Part model, mm, in its own coordinate system. A direction names the side the tool comes from. Give positions to 0.01 mm unless a question says otherwise; leave off trailing zeros. Loops run counter-clockwise (first coordinate to the right, second up) from the corner with the lowest first, then second, coordinate; pieces in that order, holes last. Notation, with made-up numbers: (80, 34.5) -> (90, 34.5) arc R12 cw to (90, 43.5) -> close; hole circle Ø8 at (-19.75, -17). An arc over 180 degrees is marked (long way). One line per question, with ' | ' between items.
```python
from build123d import *

# Parameters (mm, degrees)
PAD009_START    = 5
SKETCH014_R     = 1.4
SKETCH014_W     = 4
SKETCH014_H     = 8
SKETCH014_W_2   = 8
SKETCH014_H_2   = 4
PAD009_DEPTH    = 5
POCKET010_DEPTH = 2.5
POCKET011_DEPTH = 3
SKETCH022_R     = 2.5
POCKET012_DEPTH = 1
POCKET012_TAPER = 45


with BuildPart() as part:
    # Sketch014 → Pad009 (new body)
    with BuildSketch(Plane.XY.offset(PAD009_START)):
        with BuildLine():
            Line((-89, 43), (-89, -43))
            ThreePointArc((-89, -43), (-87.535534, -46.535534), (-84, -48))
            Line((-84, -48), (31, -48))
            ThreePointArc((31, -48), (34.535534, -46.535534), (36, -43))
            Line((36, -43), (36, 43))
            ThreePointArc((36, 43), (34.535534, 46.535534), (31, 48))
            Line((31, 48), (-84, 48))
            ThreePointArc((-84, 48), (-87.535534, 46.535534), (-89, 43))
        make_face()
        with Locations((-9, 43)):
            Circle(SKETCH014_R, mode=Mode.SUBTRACT)
        with Locations((9, 43)):
            Circle(SKETCH014_R, mode=Mode.SUBTRACT)
        with Locations((-9, -43)):
            Circle(SKETCH014_R, mode=Mode.SUBTRACT)
        with Locations((9, -43)):
            Circle(SKETCH014_R, mode=Mode.SUBTRACT)
        with Locations((-37.5, 12)):
            Circle(SKETCH014_R, mode=Mode.SUBTRACT)
        with Locations((2.5, 12)):
            Circle(SKETCH014_R, mode=Mode.SUBTRACT)
        with Locations((2.5, -12)):
            Circle(SKETCH014_R, mode=Mode.SUBTRACT)
        with Locations((-37.5, -12)):
            Circle(SKETCH014_R, mode=Mode.SUBTRACT)
        with Locations((-83.5, 15)):
            Circle(SKETCH014_R, mode=Mode.SUBTRACT)
        with Locations((-63.5, 15)):
            Circle(SKETCH014_R, mode=Mode.SUBTRACT)
        with Locations((-63.5, -15)):
            Circle(SKETCH014_R, mode=Mode.SUBTRACT)
        with Locations((-83.5, -15)):
            Circle(SKETCH014_R, mode=Mode.SUBTRACT)
        with Locations((-46.5, 24.5)):
            Circle(SKETCH014_R, mode=Mode.SUBTRACT)
        with Locations((-46.5, -24.5)):
            Circle(SKETCH014_R, mode=Mode.SUBTRACT)
        with Locations((11.5, -24.5)):
            Circle(SKETCH014_R, mode=Mode.SUBTRACT)
        with Locations((11.5, 24.5)):
            Circle(SKETCH014_R, mode=Mode.SUBTRACT)
        with BuildLine():
            Line((-9, 35), (-9, 29))
            ThreePointArc((-9, 29), (-8.707107, 28.292893), (-8, 28))
            Line((-8, 28), (8, 28))
            ThreePointArc((8, 28), (8.707107, 28.292893), (9, 29))
            Line((9, 29), (9, 35))
            ThreePointArc((9, 35), (8.707107, 35.707107), (8, 36))
            Line((8, 36), (-8, 36))
            ThreePointArc((-8, 36), (-8.707107, 35.707107), (-9, 35))
        make_face(mode=Mode.SUBTRACT)
        with BuildLine():
            Line((-9, -29), (-9, -35))
            ThreePointArc((-9, -35), (-8.707107, -35.707107), (-8, -36))
            Line((-8, -36), (8, -36))
            ThreePointArc((8, -36), (8.707107, -35.707107), (9, -35))
            Line((9, -35), (9, -29))
            ThreePointArc((9, -29), (8.707107, -28.292893), (8, -28))
            Line((8, -28), (-8, -28))
            ThreePointArc((-8, -28), (-8.707107, -28.292893), (-9, -29))
        make_face(mode=Mode.SUBTRACT)
        Polygon((28.8, 45), (28.8, 37), (21.9, 37), (21.9, 37.6), (15, 37.6), (15, 44.4), (21.9, 44.4), (21.9, 45), align=None, mode=Mode.SUBTRACT)
        with Locations((32, 29)):
            Rectangle(SKETCH014_W, SKETCH014_H, mode=Mode.SUBTRACT)
        with Locations((32, -29)):
            Rectangle(SKETCH014_W, SKETCH014_H, mode=Mode.SUBTRACT)
        with Locations((-29, 44)):
            Rectangle(SKETCH014_W_2, SKETCH014_H_2, mode=Mode.SUBTRACT)
        with Locations((-29, -44)):
            Rectangle(SKETCH014_W_2, SKETCH014_H_2, mode=Mode.SUBTRACT)
        with Locations((-85, 29)):
            Rectangle(SKETCH014_W, SKETCH014_H, mode=Mode.SUBTRACT)
        with Locations((-85, -29)):
            Rectangle(SKETCH014_W, SKETCH014_H, mode=Mode.SUBTRACT)
    extrude(amount=PAD009_DEPTH)

    # Sketch020 (on Face73 of Pad009) → Pocket010 (cut)
    with BuildSketch(Plane(origin=(0, 0, 5), x_dir=(1, 0, 0), z_dir=(0, 0, -1))):
        Polygon((-46.5, -27.5), (-43.901924, -26), (-43.901924, -23), (-46.5, -21.5), (-49.098076, -23), (-49.098076, -26), align=None)
        Polygon((-46.5, 27.5), (-49.098076, 26), (-49.098076, 23), (-46.5, 21.5), (-43.901924, 23), (-43.901924, 26), align=None)
        Polygon((11.5, 27.5), (8.901924, 26), (8.901924, 23), (11.5, 21.5), (14.098076, 23), (14.098076, 26), align=None)
        Polygon((11.5, -27.5), (14.098076, -26), (14.098076, -23), (11.5, -21.5), (8.901924, -23), (8.901924, -26), align=None)
    extrude(amount=-POCKET010_DEPTH, mode=Mode.SUBTRACT)

    # Sketch021 (on Face5 of Pocket010) → Pocket011 (cut)
    with BuildSketch(Plane.XY.offset(10)):
        Polygon((-83.5, 12), (-80.901924, 13.5), (-80.901924, 16.5), (-83.5, 18), (-86.098076, 16.5), (-86.098076, 13.5), align=None)
        Polygon((-83.5, -18), (-80.901924, -16.5), (-80.901924, -13.5), (-83.5, -12), (-86.098076, -13.5), (-86.098076, -16.5), align=None)
        Polygon((-63.5, 12), (-60.901924, 13.5), (-60.901924, 16.5), (-63.5, 18), (-66.098076, 16.5), (-66.098076, 13.5), align=None)
        Polygon((-63.5, -12), (-66.098076, -13.5), (-66.098076, -16.5), (-63.5, -18), (-60.901924, -16.5), (-60.901924, -13.5), align=None)
        Polygon((-37.5, -15), (-34.901924, -13.5), (-34.901924, -10.5), (-37.5, -9), (-40.098076, -10.5), (-40.098076, -13.5), align=None)
        Polygon((-37.5, 15), (-40.098076, 13.5), (-40.098076, 10.5), (-37.5, 9), (-34.901924, 10.5), (-34.901924, 13.5), align=None)
        Polygon((2.5, 15), (-0.098076, 13.5), (-0.098076, 10.5), (2.5, 9), (5.098076, 10.5), (5.098076, 13.5), align=None)
        Polygon((2.5, -15), (5.098076, -13.5), (5.098076, -10.5), (2.5, -9), (-0.098076, -10.5), (-0.098076, -13.5), align=None)
    extrude(amount=-POCKET011_DEPTH, mode=Mode.SUBTRACT)

    # Sketch022 (on Face5 of Pocket011) → Pocket012 (cut)
    with BuildSketch(Plane.XY.offset(10)):
        with Locations((-9, 43)):
            Circle(SKETCH022_R)
        with Locations((9, 43)):
            Circle(SKETCH022_R)
        with Locations((-9, -43)):
            Circle(SKETCH022_R)
        with Locations((9, -43)):
            Circle(SKETCH022_R)
    extrude(amount=-POCKET012_DEPTH, taper=POCKET012_TAPER, mode=Mode.SUBTRACT)


solid = part.part
```
1) Saw through at B-B (x = -3). Give the cut face in (y, z).
Found:
outline: (-48, 5) -> (-36, 5) -> (-36, 10) -> (-48, 10) -> close; (-28, 5) -> (28, 5) -> (28, 10) -> (-28, 10) -> close; (36, 5) -> (48, 5) -> (48, 10) -> (36, 10) -> close
2) Pin check, flat tips, straight feed: P1, Ø2.5, axis at x = -83, y = -15.5, coming from the +Z side; P2, Ø3.5, axis at x = 11.5, y = 24.5, coming from the -Z side; P3, Ø3, axis at x = -84.5, z = 7, coming from the +Y side; P4, Ø3.5, axis at x = 9, y = -42.5, coming from the +Z side. Stop position of each tip, or through.
Found:
P1: z = 7 | P2: z = 7.5 | P3: y = 48 | P4: z = 9.75
3) Tool access for faces 1 (the flat face through (-47.82, -22.26, 6.23)), 2 (the flat face through (1.22, 14.26, 8.52)), 3 (the flat face through (34, -29, 7)): list every direction of +Z, -Z, +X, -X, +Y, -Y with a clear straight run to the whole face (end or side of a thin tool).
Found:
face 1: -Z | face 2: +Z | face 3: +Z, -Z
4) Saw through at A-A (x = -27.5). Give the cut face in (y, z).
Found:
outline: (-48, 5) -> (-46, 5) -> (-46, 10) -> (-48, 10) -> close; (-42, 5) -> (42, 5) -> (42, 10) -> (-42, 10) -> close; (46, 5) -> (48, 5) -> (48, 10) -> (46, 10) -> close
5) Drill centre lines: line 1 (Y direction, x = 4.5, z = 6.7); line 2 (X direction, y = -12, z = 6.2); line 3 (Y direction, x = -63.5, z = 5.85). Where is each one in solid material? Low to high.
Found:
line 1: -48 to -36, -28 to 28, 36 to 48 | line 2: -89 to -38.9, -36.1 to 1.1, 3.9 to 36 | line 3: -48 to -16.4, -13.6 to 13.6, 16.4 to 48
